Design review of the part shown in the three views and the two pictorial views. Dimensions are in mm from the part's minimum x, y and z. Round coordinates to 2 decimals unless told otherwise and drop trailing zeros. Order: outer loops, then holes, each group sorted by start corner. A loop starts at its lowest first (then second) coordinate and runs counter-clockwise, first axis right, second up.
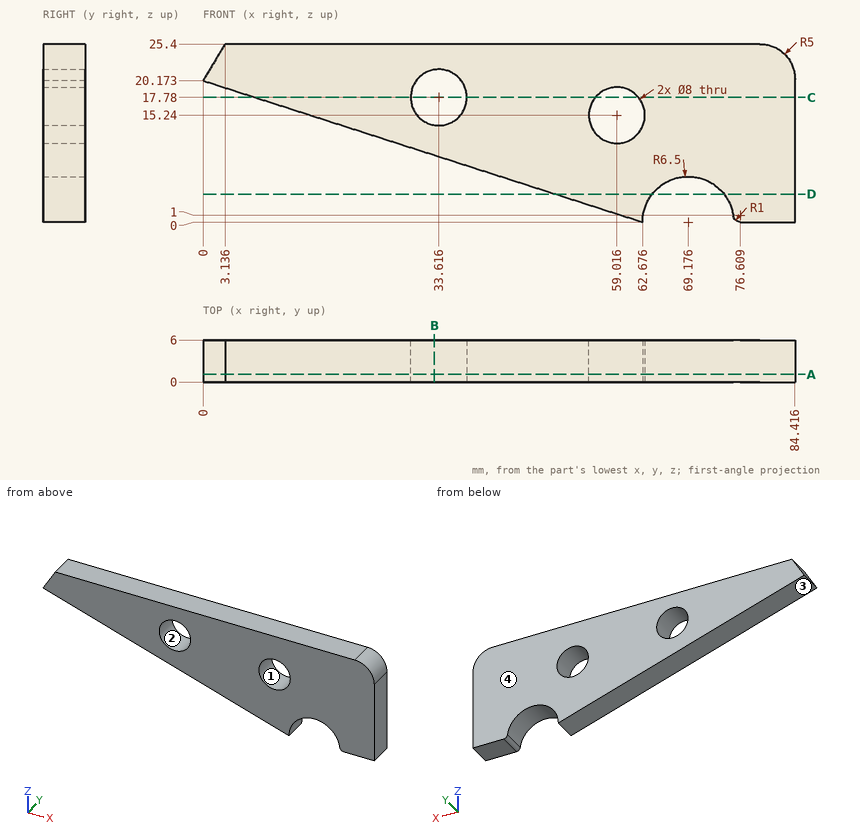
1) Take a section at A-A on y = 1.1. Give the boundary of the cut face in (x, z).
Results:
outline: (0, 20.17) - (62.68, 0) arc R6.5 cw to (75.62, 0.87) arc R1 ccw to (76.61, 0) - (84.42, 0) - (84.42, 20.4) arc R5 ccw to (79.42, 25.4) - (3.14, 25.4) - close; hole circle Ø8 at (33.62, 17.78); hole circle Ø8 at (59.02, 15.24)
2) To check wall thickness, follow line 1 along Z through (x, y) = (65.5, 3); line 2 along X through (y, z) = (0.6, 24.25) (1 decimal); line 3 along Z through (x, y) = (76, 1.25) (1 decimal). State the ranges of each line that lie inside material, in increasing order.
Results:
line 1: z = 5.36 to 25.4
line 2: x = 2.4 to 82.6
line 3: z = 0.2 to 25.4
3) Take a section at B-B on x = 33. Give the boundary of the cut face in (y, z).
Results:
outline: (0, 9.55) - (6, 9.55) - (6, 13.83) - (0, 13.83) - close; (0, 21.73) - (6, 21.73) - (6, 25.4) - (0, 25.4) - close
4) Take a section at C-C on z = 17.78. Give the boundary of the cut face in (x, y), plus the area to 3 significant figures.
Results:
outline: (7.43, 0) - (29.62, 0) - (29.62, 6) - (7.43, 6) - close; (37.62, 0) - (55.93, 0) - (55.93, 6) - (37.62, 6) - close; (62.11, 0) - (84.42, 0) - (84.42, 6) - (62.11, 6) - close
area: 377 mm2
5) Take a section at D-D on z = 4. Give the boundary of the cut face in (x, y).
Results:
outline: (50.25, 0) - (64.05, 0) - (64.05, 6) - (50.25, 6) - close; (74.3, 0) - (84.42, 0) - (84.42, 6) - (74.3, 6) - close
6) The part is to be moulded in two halves that separate along X. For the marked faces 1, 2, 3 and 4, say which applies: released by +X, released by -X, zero draft, split by the parting line, or undercut.
Results:
face 1: undercut
face 2: undercut
face 3: released by -X
face 4: zero draft
